Geometry: final body of the model. Coordinates: model frame, mm. Face numbers are marked on the shaded views. A direction names the side the tool comes from. Give positions to 0.01 mm unless a question says otherwise; leave off trailing zeros. Write each loop counter-clockwise with the first axis right and the second up, starting at its lowest first coordinate (ties: lowest second). Pieces come first, ordered by that corner, then holes. Notation, with made-up numbers: (7.5, 8) -> (31.5, 8) arc R6 cw to (31.5, 16) -> close; hole circle Ø9 at (59, -24.75). An arc over 180 degrees is marked (long way). Answer in a Markdown table with one row per item. Add a question column.
Item 1: First-contact query: P1, Ø1.5, axis at x = -1.5, z = 1, coming from the +Y side. Flat tip, straight axial feed; report the tip coordinate or a pass-through.
Item 2: Access query for the marked faces 1, 2 and 3. Directions: +Z, -Z, +X, -X, +Y, -Y. A direction counts if a zero-diameter tool reaches every point of the face in a straight line with its end or side. Return the directions, or none.
Item 3: Section query B-B on x = 0. Output: boundary loops of the cut face in (y, z).
Item 4: Material intervals for probe 1 along Y at (x, z) = (-0.4, -1.35); probe 2 along Z at (x, y) = (-0.1, 1), sorted ascending. Write a range as from..to.
Item 5: Section query D-D on y = 6.25. Output: boundary loops of the cut face in (x, z).
Item 6: Section query A-A on z = 0. Output: boundary loops of the cut face in (x, y).
Item 7: Section query C-C on y = -2. Output: boundary loops of the cut face in (x, z).
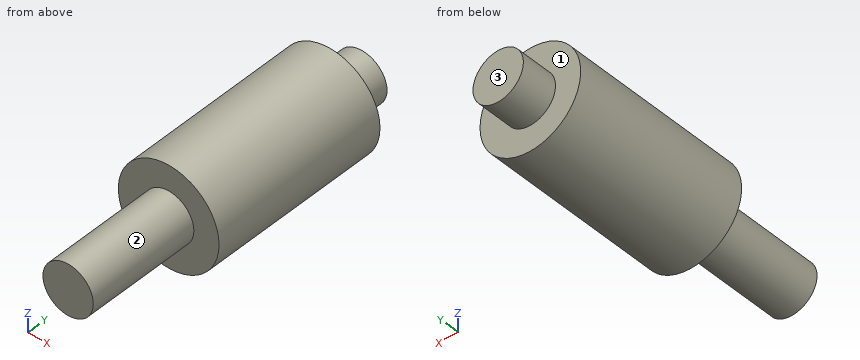
```python
from build123d import *

# Parameters (mm, degrees)
SKETCH1_R           = 2.2
BOSS_EXTRUDE1_DEPTH = 8
SKETCH2_R           = 1.1
BOSS_EXTRUDE2_DEPTH = 1.6
SKETCH3_R           = 1.1
BOSS_EXTRUDE3_DEPTH = 5


with BuildPart() as part:
    # Sketch1 → Boss-Extrude1 (new body)
    with BuildSketch(Plane(origin=(0, 0, 0), x_dir=(1, 0, 0), z_dir=(0, 1, 0))):
        Circle(SKETCH1_R)
    extrude(amount=BOSS_EXTRUDE1_DEPTH)

    # Sketch2 → Boss-Extrude2 (add)
    with BuildSketch(Plane(origin=(0, 8, 0), x_dir=(1, 0, 0), z_dir=(0, 1, 0))):
        Circle(SKETCH2_R)
    extrude(amount=BOSS_EXTRUDE2_DEPTH)

    # Sketch3 → Boss-Extrude3 (add)
    with BuildSketch(Plane.XZ):
        Circle(SKETCH3_R)
    extrude(amount=BOSS_EXTRUDE3_DEPTH)


solid = part.part
```
Findings below:
| question | item | result |
|---|---|---|
| 1 | P1 | stops at y = 9.6 |
| 2 | face 1 | +Y |
| 2 | face 2 | -Y |
| 2 | face 3 | +Z, -Z, +X, -X, +Y |
| 3 | outline | (-5, -1.1) -> (0, -1.1) -> (0, -2.2) -> (8, -2.2) -> (8, -1.1) -> (9.6, -1.1) -> (9.6, 1.1) -> (8, 1.1) -> (8, 2.2) -> (0, 2.2) -> (0, 1.1) -> (-5, 1.1) -> close |
| 4 | probe 1 | y = 0..8 |
| 4 | probe 2 | z = -2.2..2.2 |
| 5 | outline | circle Ø4.4 at (0, 0) |
| 6 | outline | (-2.2, 0) -> (-1.1, 0) -> (-1.1, -5) -> (1.1, -5) -> (1.1, 0) -> (2.2, 0) -> (2.2, 8) -> (1.1, 8) -> (1.1, 9.6) -> (-1.1, 9.6) -> (-1.1, 8) -> (-2.2, 8) -> close |
| 7 | outline | circle Ø2.2 at (0, 0) |
